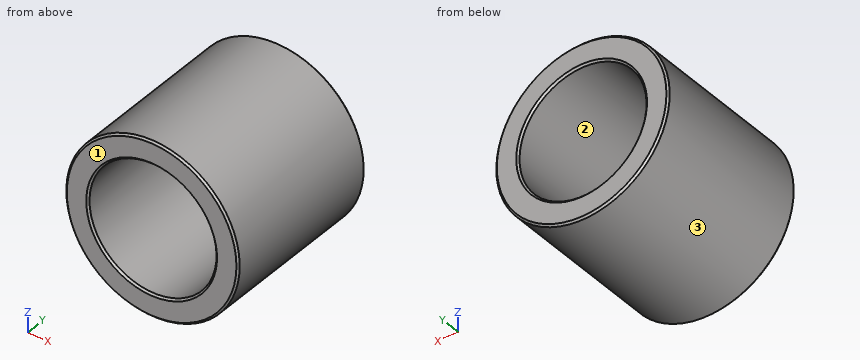
from build123d import *

# Parameters (mm, degrees)
SKETCH1_R           = 32.5
BOSS_EXTRUDE1_DEPTH = 63.607411
SKETCH2_R           = 23.815414931
CUT_EXTRUDE1_DEPTH  = 79.475491296
CHAMFER1_SIZE       = 0.70101
CHAMFER1_SIZE_2     = 0.698911


with BuildPart() as part:
    # Sketch1 → Boss-Extrude1 (new body)
    with BuildSketch(Plane(origin=(0, 0, 0), x_dir=(1, 0, 0), z_dir=(0, 1, 0))):
        with Locations(Location((0, 0, 0), (0, 0, 270))):
            Circle(SKETCH1_R)
    extrude(amount=BOSS_EXTRUDE1_DEPTH)

    # Sketch2 → Cut-Extrude1 (cut, through all)
    with BuildSketch(Plane(origin=(0, 0, 0), x_dir=(1, 0, 0), z_dir=(0, 1, 0))):
        with Locations(Location((0, 0, 0), (0, 0, 270))):
            Circle(SKETCH2_R)
    extrude(amount=CUT_EXTRUDE1_DEPTH, mode=Mode.SUBTRACT)

    # Chamfer1
    # the kernel refuses this chamfer: 0.70101, 0.698911 mm, written as the material it takes off along each edge
    with BuildSketch(Plane(origin=(0, 0, 0), x_dir=(0, 0, 1), z_dir=(-1, 0, 0))) as chamfer1_piece_1:
        Polygon((32.5, CHAMFER1_SIZE), (32.5 - CHAMFER1_SIZE_2, 0), (32.5, 0), align=None)
    revolve(axis=Axis((0, 0, 0), (0, 1, 0)), mode=Mode.SUBTRACT)
    with BuildSketch(Plane(origin=(0, 63.607411, 0), x_dir=(0, 0, 1), z_dir=(-1, 0, 0))) as chamfer1_piece_2:
        Polygon((32.5, -CHAMFER1_SIZE_2), (32.5 - CHAMFER1_SIZE, 0), (32.5, 0), align=None)
    revolve(axis=Axis((0, 63.607411, 0), (0, 1, 0)), mode=Mode.SUBTRACT)
    with BuildSketch(Plane(origin=(0, 0, 0), x_dir=(0, 0, 1), z_dir=(-1, 0, 0))) as chamfer1_piece_3:
        Polygon((23.815414931 + CHAMFER1_SIZE, 0), (23.815414931, CHAMFER1_SIZE_2), (23.815414931, 0), align=None)
    revolve(axis=Axis((0, 0, 0), (0, 1, 0)), mode=Mode.SUBTRACT)
    with BuildSketch(Plane(origin=(0, 63.607411, 0), x_dir=(0, 0, 1), z_dir=(1, 0, 0))) as chamfer1_piece_4:
        Polygon((23.815414931 + CHAMFER1_SIZE_2, 0), (23.815414931, CHAMFER1_SIZE), (23.815414931, 0), align=None)
    revolve(axis=Axis((0, 63.607411, 0), (0, -1, 0)), mode=Mode.SUBTRACT)


solid = part.part
Read the model definition and answer for the solid it produces. Units are mm, in the model's axes. Face numbers are marked on the shaded views. Give positions to 0.01 mm unless a question says otherwise; leave off trailing zeros. Loops run counter-clockwise (first coordinate to the right, second up) from the corner with the lowest first, then second, coordinate; pieces in that order, holes last. Notation, with made-up numbers: (21.5, 75.25) -> (76.5, 75.25) arc R21 ccw to (76.5, 89.25) -> close; hole circle Ø8 at (41.5, -36). An arc over 180 degrees is marked (long way). Answer as CSV lines item,"result".
Item 1: Determine the mould class of the marked faces 1, 2 and 3 for opening direction Z: +Z half, -Z half, draft (parallel to the pull), parting line (faces both ways), or undercut.
Returned:
face 1,"draft"
face 2,"undercut"
face 3,"parting line"
Item 2: Each of these flat-tipped pins is pushed along its axis until it touches: pin 1 (8 mm diameter, centred on y = 9, z = 17.5, fed in from -X); pin 2 (5 mm diameter, centred on y = 39.5, z = -1, fed in from +X); pin 3 (2 mm diameter, centred on x = 14, y = 14.5, fed in from +Z); pin 4 (12 mm diameter, centred on x = 21, z = 7, fed in from +Y). Where does it stop, or does it pass through?
Returned:
pin 1,"stops at x = -29.56"
pin 2,"stops at x = 32.5"
pin 3,"stops at z = 29.79"
pin 4,"stops at y = 63.61"
Item 3: Find section A-A on x = 0. Give the vertices of the cut face in (y, z).
Returned:
outline,"(0, -31.8) -> (0.7, -32.5) -> (62.91, -32.5) -> (63.61, -31.8) -> (63.61, -24.51) -> (62.91, -23.82) -> (0.7, -23.82) -> (0, -24.52) -> close; (0, 24.52) -> (0.7, 23.82) -> (62.91, 23.82) -> (63.61, 24.51) -> (63.61, 31.8) -> (62.91, 32.5) -> (0.7, 32.5) -> (0, 31.8) -> close"
Item 4: Find section C-C on y = 9. Give the vertices of the cut face in (x, z), plus the area to 3 significant figures.
Returned:
outline,"circle Ø65 at (0, 0); hole circle Ø47.63 at (0, 0)"
area,"1,540 mm²"
Item 5: Find section B-B on z = 0. Give the vertices of the cut face in (x, y).
Returned:
outline,"(-32.5, 0.7) -> (-31.8, 0) -> (-24.52, 0) -> (-23.82, 0.7) -> (-23.82, 62.91) -> (-24.51, 63.61) -> (-31.8, 63.61) -> (-32.5, 62.91) -> close; (23.82, 0.7) -> (24.52, 0) -> (31.8, 0) -> (32.5, 0.7) -> (32.5, 62.91) -> (31.8, 63.61) -> (24.51, 63.61) -> (23.82, 62.91) -> close"
Item 6: Consider line 1 (X direction, y = 35, z = 0); line 2 (Z direction, x = 12.5, y = 9); line 3 (Z direction, x = 1.5, y = 39). Determine where each line is inside the solid, lowest interval first. Write a range as [from, to].
Returned:
line 1,"x = [-32.5, -23.82], [23.82, 32.5]"
line 2,"z = [-30, -20.27], [20.27, 30]"
line 3,"z = [-32.47, -23.77], [23.77, 32.47]"
